Model file for the job. Use its own axes, mm. Face numbers are marked on the shaded views. A direction names the side the tool comes from. Coordinates: 2 decimals unless noted, no trailing zeros. Put each result on its own line as item: value. Start each with the question number.
```python
from build123d import *

# Parameters (mm, degrees)
BOSS_EXTRUDE1_START = 1
SKETCH2_R           = 0.75
BOSS_EXTRUDE1_DEPTH = 1
CHAMFER1_SIZE       = 0.5


with BuildPart() as part:
    # Sketch1 → Revolve1 (revolve)
    with BuildSketch(Plane(origin=(0, 0, 0), x_dir=(0, 0, -1), z_dir=(1, 0, 0)), mode=Mode.PRIVATE) as revolve1_sk:
        with BuildLine():
            Line((87.5, 6), (76.15, 6))
            Line((76.15, 6), (76.15, 5.75))
            Line((76.15, 5.75), (75, 5.75))
            Line((75, 5.75), (75, 14.7))
            ThreePointArc((75, 14.7), (0, 15), (-75, 14.7))
            Line((-75, 14.7), (-75, 5.75))
            Line((-75, 5.75), (-76.15, 5.75))
            Line((-76.15, 5.75), (-76.15, 6))
            Line((-76.15, 6), (-87.5, 6))
            Line((-87.5, 6), (-87.5, 0))
            Line((-87.5, 0), (87.5, 0))
            Line((87.5, 0), (87.5, 6))
        make_face()
    revolve(revolve1_sk.sketch.rotate(Axis((0, 0, 87.5), (0, 0, -1)), 180), axis=Axis((0, 0, 87.5), (0, 0, -1)))

    # Sketch2 → Boss-Extrude1 (add)
    with BuildSketch(Plane.XY.offset(75).offset(BOSS_EXTRUDE1_START)):
        with BuildLine():
            Line((-0.45, -8.95), (-0.45, -5.732364259))
            ThreePointArc((-0.45, -5.732364259), (0, 5.75), (0.45, -5.732364259))
            Line((0.45, -5.732364259), (0.45, -8.95))
            Line((0.45, -8.95), (2.25, -8.95))
            ThreePointArc((2.25, -8.95), (3.452081528, -8.452081528), (3.95, -7.25))
            Line((3.95, -7.25), (3.95, -6.512622113))
            ThreePointArc((3.95, -6.512622113), (4.117151006, -5.777520785), (4.585734072, -5.186975842))
            ThreePointArc((4.585734072, -5.186975842), (0, 7.85), (-4.585734072, -5.186975842))
            ThreePointArc((-4.585734072, -5.186975842), (-4.117151006, -5.777520785), (-3.95, -6.512622113))
            Line((-3.95, -6.512622113), (-3.95, -7.25))
            ThreePointArc((-3.95, -7.25), (-3.452081528, -8.452081528), (-2.25, -8.95))
            Line((-2.25, -8.95), (-0.45, -8.95))
        make_face()
        with Locations((-2.2, -7.25)):
            Circle(SKETCH2_R, mode=Mode.SUBTRACT)
        with Locations((2.2, -7.25)):
            Circle(SKETCH2_R, mode=Mode.SUBTRACT)
    boss_extrude1 = extrude(amount=-BOSS_EXTRUDE1_DEPTH)

    # Mirror1: Boss-Extrude1 across plane
    add(boss_extrude1.mirror(Plane.XY))

    # Chamfer1
    chamfer1_edges = [part.edges().sort_by_distance(p)[0] for p in [
        (0, 6, 87.5),
        (0, 6, -87.5),
    ]]
    chamfer(chamfer1_edges, length=CHAMFER1_SIZE)


solid = part.part
```
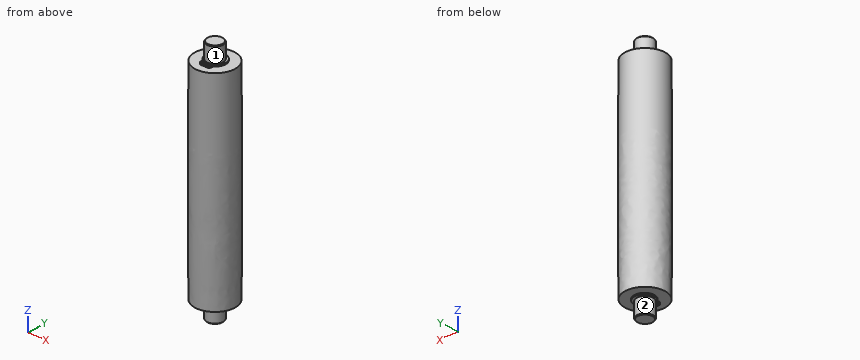
Item 1: Wall check: line 1 along Z through (x, y) = (-7.5, -9); line 2 along Y through (x, z) = (2.2, 75.75); line 3 along Y through (x, z) = (5, 33). Give the ranges that are in metal, low to high.
Item 2: 3-axis set-ups, long thin cutter, end or side, ignore diameter. For the marked faces 1 and 2: which of +Z, -Z, +X, -X, +Y, -Y reach the whole face in a straight line?
Item 3: Flat gauge pins, fed straight in: pin 1 Ø6 at (x, y) = (7, 7) entering from +Z; pin 2 Ø0.8 at (x, y) = (2.5, -7) entering from -Z; pin 3 Ø5 at (y, z) = (-5.5, -1.5) entering from +X. Where does each tip first touch, or does it go through?
Here are the results:
1. line 1: z = -75 to 75
1. line 2: y = -8.95 to -8, -6.5 to 7.51
1. line 3: y = -14.08 to 14.08
2. face 1: +Z
2. face 2: -Z
3. pin 1: stops at z = 76
3. pin 2: stops at z = -76
3. pin 3: stops at x = 14.7
